The listing builds one solid part. Answer for the finished solid, in the listing's coordinates (mm). A direction names the side the tool comes from. Coordinates: 2 decimals unless noted, no trailing zeros. Order: outer loops, then holes, each group sorted by start corner. A loop starts at its lowest first (then second) coordinate and runs counter-clockwise, first axis right, second up. Notation, with made-up numbers: (38.25, 44) - (42.25, 44) arc R13 cw to (42.25, 68) - close; hole circle Ø1 at (-31.75, 3.5). An arc over 180 degrees is marked (long way). Use a Markdown table: item, result. Add a question column.
Item 1: For faces 5 (the flat face through (63.2, -1, -9)), 6 (the flat face through (32.704, 6.194, -25.478)), 7 (the flat face through (64.993, 9.056, -22.683)), 8 (the flat face through (65, -1, -11.347)), determine the directions among +Z, -Z, +X, -X, +Y, -Y from which every point of the face is accessible in a straight line to the end or side of a thin tool.
Item 2: Find the intervals of material crossed by line 1 along Z through (x, y) = (12.2, 1.5); line 2 along X through (y, z) = (-1.5, -24); line 3 along Z through (x, y) = (61, -1.75), in increasing order.
Item 3: A flat-ended cylindrical pin translates along its axis: P1, Ø5.5, axis at x = 41, z = -12.5, coming from the -Y side. Find the tip coordinate at first contact, or state that the pin passes through.
Item 4: The part is cut by section D-D, the plane z = -18.5. Give the vertices of the cut face in (x, y).
Item 5: The part is cut by section A-A, the plane y = 12.25. Give the vertices of the cut face in (x, z), then the cut area to 3 significant figures.
Item 6: The part is cut by section B-B, the plane z = -8.5. Give the vertices of the cut face in (x, y) (3 decimals).
Item 7: The mould has two halves that part along Y. Classify faces 1 (the flat face through (1.257, 9.056, -22.683)), 2 (the flat face through (33, -3.175, -32)), 3 (the flat face through (3.05, -1, -9)), 4 (the flat face through (33, 19.284, -5)): released by +Y, released by -Y, zero draft, split by the parting line, or undercut.
from build123d import *
from OCP.BRepFilletAPI import BRepFilletAPI_MakeChamfer

# Parameters (mm, degrees)
BOSS_EXTRUDE1_DEPTH = 66.25
BOSS_EXTRUDE2_DEPTH = 3.05
BOSS_EXTRUDE3_DEPTH = 3.175
SKETCH2_4_R         = 1.5
CUT_EXTRUDE1_DEPTH  = 3
CHAMFER1_SIZE       = 1.5
CHAMFER3_SIZE       = 2.675
CHAMFER4_SIZE       = 0.5
CHAMFER4_SIZE_2     = 0.353553391


with BuildPart() as part:
    # Sketch1 → Boss-Extrude1 (new body)
    with BuildSketch(Plane(origin=(0, 0, 0), x_dir=(0, 0, -1), z_dir=(1, 0, 0))):
        Polygon((14.843681451, 19.28355698), (34.843681451, 19.28355698), (34.843681451, 0), (0, 0), (0, 19.28355698), (10, 19.28355698), (24.28355698, 5), (26.705397706, 7.421840726), align=None)
    extrude(amount=BOSS_EXTRUDE1_DEPTH)

    # Sketch1<4> → Boss-Extrude2 (add)
    with BuildSketch(Plane(origin=(0, 0, 0), x_dir=(0, 0, -1), z_dir=(1, 0, 0))):
        Polygon((23.876970581, 10.25026785), (21.455129855, 7.828427125), (24.28355698, 5), (26.705397706, 7.421840726), align=None)
    boss_extrude2 = extrude(amount=BOSS_EXTRUDE2_DEPTH)

    # Mirror1: Boss-Extrude2 across plane
    add(boss_extrude2.mirror(Plane.ZY.offset(-33.125)))

    # Sketch2 → Boss-Extrude3 (add)
    with BuildSketch(Plane(origin=(0, 0, 0), x_dir=(1, 0, 0), z_dir=(0, 1, 0))):
        Polygon((0, 11.346840726), (0, 0), (66.25, 0), (66.25, 11.346840726), (63.2, 11.346840726), (63.2, 7.246840726), (3.05, 7.246840726), (3.05, 11.346840726), align=None)
        Polygon((0, 34.843681451), (0, 19.446840726), (3.05, 19.446840726), (3.05, 27.596840726), (63.2, 27.596840726), (63.2, 19.446840726), (66.25, 19.446840726), (66.25, 34.843681451), align=None)
    extrude(amount=-BOSS_EXTRUDE3_DEPTH)

    # Sketch2<4> → Cut-Extrude1 (cut)
    with BuildSketch(Plane(origin=(0, 0, 0), x_dir=(1, 0, 0), z_dir=(0, 1, 0))):
        with Locations(Location((54.05, 14.246840726, 0), (0, 0, 90))):
            Circle(SKETCH2_4_R)
        with Locations(Location((12.2, 14.246840726, 0), (0, 0, 90))):
            Circle(SKETCH2_4_R)
    extrude(amount=CUT_EXTRUDE1_DEPTH, mode=Mode.SUBTRACT)

    # Chamfer1
    chamfer1_edges = [part.edges().sort_by_distance(p)[0] for p in [
        (54.05, 3, -12.746840726),
        (54.05, 0, -12.746840726),
        (12.2, 0, -12.746840726),
        (12.2, 3, -12.746840726),
    ]]
    chamfer(chamfer1_edges, length=CHAMFER1_SIZE - 0.0001)  # a hair under: the kernel refuses the full size

    # Chamfer3
    chamfer3_edges = [part.edges().sort_by_distance(p)[0] for p in [
        (33.125, 0, -27.596840726),
    ]]
    chamfer(chamfer3_edges, length=CHAMFER3_SIZE)

    # Chamfer4
    chamfer4_edges_1 = [part.edges().sort_by_distance(p)[0] for p in [
        (3.05, 9.039347488, -22.666050218),
        (63.2, 9.039347488, -22.666050218),
        (3.05, -3.175, -23.521840726),
        (1.525, -3.175, -19.446840726),
        (63.2, -3.175, -23.521840726),
        (64.725, -3.175, -19.446840726),
        (1.525, -3.175, -11.346840726),
        (3.05, -3.175, -9.296840726),
        (33.125, -3.175, -7.246840726),
        (63.2, -3.175, -9.296840726),
        (64.725, -3.175, -11.346840726),
        (33.125, -3.175, -27.596840726),
    ]]
    chamfer4_edges_2 = [part.edges().sort_by_distance(p)[0] for p in [
        (33.125, 19.28355698, -14.843681451),
    ]]
    chamfer4_side_2 = [part.faces().sort_by_distance(p)[0] for p in [
        (33.125, 19.28355698, -14.850752519),
    ]]
    chamfer4 = BRepFilletAPI_MakeChamfer(part.part.solid().wrapped)
    for e in chamfer4_edges_1:
        chamfer4.Add(CHAMFER4_SIZE - 0.0001, e.wrapped)
    for e in chamfer4_edges_2:
        chamfer4.Add(CHAMFER4_SIZE - 0.0001, CHAMFER4_SIZE_2 - 0.0001, e.wrapped, chamfer4_side_2[0].wrapped)
    add(Compound.cast(chamfer4.Shape()), mode=Mode.REPLACE)  # a hair under: the kernel refuses the full size


solid = part.part
Solution:
| question | item | result |
|---|---|---|
| 1 | face 5 | -Y |
| 1 | face 6 | none |
| 1 | face 7 | +X, -X |
| 1 | face 8 | +X, -X, -Y |
| 2 | line 1 | z = -34.84 to -15.75, -12.75 to 0 |
| 2 | line 2 | x = 0 to 3.05, 63.2 to 66.25 |
| 2 | line 3 | z = -34.84 to -26.67, -7.25 to 0 |
| 3 | P1 | stops at y = 0 |
| 4 | outline | (0, 0) - (66.25, 0) - (66.25, 10.78) - (0, 10.78) - close; (0, 15.63) - (66.25, 15.63) - (66.25, 19.28) - (0, 19.28) - close |
| 5 | outline | (0, -34.84) - (66.25, -34.84) - (66.25, -21.88) - (0, -21.88) - close; (0, -17.03) - (66.25, -17.03) - (66.25, 0) - (0, 0) - close |
| 5 | area | 1,990 mm2 |
| 6 | outline | (0, -3.175) - (2.55, -3.175) - (3.05, -2.675) - (3.05, 0) - (63.2, 0) - (63.2, -2.675) - (63.7, -3.175) - (66.25, -3.175) - (66.25, 19.284) - (0, 19.284) - close |
| 7 | face 1 | undercut |
| 7 | face 2 | released by -Y |
| 7 | face 3 | zero draft |
| 7 | face 4 | released by +Y |
